Geometry: final body of the model. Coordinates: model frame, mm. A direction names the side the tool comes from. Round coordinates to 2 decimals unless told otherwise and drop trailing zeros. Loops run counter-clockwise (first coordinate to the right, second up) from the corner with the lowest first, then second, coordinate; pieces in that order, holes last. Notation, with made-up numbers: M -5,89.25 L 49,89.25 A20 ccw 49,122.25 Z; hole C 71.25,-36 d7. An arc over 180 degrees is marked long. Answer as a JSON object with one key per item and string values.
Autodesk Inventor part; units mm, degrees
ref_plane "YZ Plane" through (0, 0, 0) normal (1, 0, 0) x (0, 1, 0)
ref_plane "XZ Plane" through (0, 0, 0) normal (0, 1, 0) x (-1, 0, 0)
ref_plane "XY Plane" through (0, 0, 0) normal (0, 0, 1) x (1, 0, 0)
sketch "Sketch1" plane through (0, 0, 0) normal (0, 0, 1) x (1, 0, 0)
  line L0 (0, 0) -> (10, 0)
  line L1 (10, 0) -> (10, 10)
  line L2 (10, 10) -> (0, 10)
  line L3 (0, 10) -> (0, 0)
  dimension "d0" = 10
  dimension "d1" = 10
extrude "Extrusion1" add sketch "Sketch1" along normal blind 1
sketch "Sketch2" plane through (0, 0, 1) normal (0, 0, 1) x (1, 0, 0)
  line L0 (10, 10) -> (0, 10)
  line L1 (5, 10) -> (5, 5)
  circle A0 centre (5, 5) radius 3.25
  point P0 (0, 0)
  dimension "d4" = 5
  dimension "d5" = 6.5
extrude "Extrusion2" add sketch "Sketch2" along normal blind 0.5
sketch "Sketch3" plane through (5, 5, 1.5) normal (0, 0, 1) x (1, 0, 0)
  circle A0 centre (0, 0) radius 3
  point P0 (-5, -5)
  dimension "d8" = 6
extrude "Extrusion3" add sketch "Sketch3" along normal blind 0.5
sketch "Sketch4" plane through (5, 5, 2) normal (0, 0, 1) x (1, 0, 0)
  line L0 (1, 0) -> (1, 1)
  line L1 (1, 1) -> (-1, 1)
  line L2 (-1, 1) -> (-1, -1)
  line L3 (-1, -1) -> (1, -1)
  line L4 (1, -1) -> (1, 0)
  point P0 (-5, -5)
  dimension "d12" = 1
  dimension "d13" = 2
  dimension "d14" = 2
extrude "Extrusion4" add sketch "Sketch4" along normal blind 2.5
sketch "Sketch5" plane through (0, 0, 1) normal (0, 0, 1) x (1, 0, 0)
  point P0 (0, 0)
sketch "Sketch6" plane through (5, 5, 4.5) normal (0, 0, 1) x (1, 0, 0)
  point P0 (-5, -5)
properties part number "BTN_2"
1) Pin query (flat end, axial travel): P1, Ø1.6, axis at x = 4.5, z = 2.5, coming from the -Y side; P2, Ø1, axis at y = 5.5, z = 3, coming from the -X side; P3, Ø4, axis at x = 2, y = 8.5, coming from the +Z side. Return the tip coordinate at first contact, or that it passes through.
Results:
{"P1": "y = 2", "P2": "x = 4", "P3": "z = 2"}
2) Ray query, line 1 (Z direction, x = 0.5, y = 7.25); line 2 (Z direction, x = 6.5, y = 4.5); line 3 (X direction, y = 4.75, z = 2.1). Return the intervals inside material, ascending.
Results:
{"line 1": "0 to 1", "line 2": "0 to 2", "line 3": "4 to 6"}
3) Section query A-A (y = 5). Return the cut outline in (x, z), and give its area (4 significant figures).
Results:
{"outline": "M 0,0 L 10,0 L 10,1 L 8.25,1 L 8.25,1.5 L 8,1.5 L 8,2 L 6,2 L 6,4.5 L 4,4.5 L 4,2 L 2,2 L 2,1.5 L 1.75,1.5 L 1.75,1 L 0,1 Z", "area": "21.25 mm2"}
4) Reachability of faces 1 (the flat face through (6, 5, 3)), 2 (the flat face through (5, 4, 3)), 3 (the flat face through (4, 5, 3)), 4 (the flat face through (1.6, 5.1, 1)) from +Z, -Z, +X, -X, +Y, -Y: full face, straight path, thin tool, end or side. Return the list, or none.
Results:
{"face 1": "+Z, +X, +Y, -Y", "face 2": "+Z, +X, -X, -Y", "face 3": "+Z, -X, +Y, -Y", "face 4": "+Z"}
5) Section query C-C (z = 4.05). Return the cut outline in (x, y).
Results:
{"outline": "M 4,4 L 6,4 L 6,6 L 4,6 Z"}
6) Section query D-D (x = 3.5). Return the cut outline in (y, z), and give its area (3 significant figures).
Results:
{"outline": "M 0,0 L 10,0 L 10,1 L 7.88,1 L 7.88,1.5 L 7.6,1.5 L 7.6,2 L 2.4,2 L 2.4,1.5 L 2.12,1.5 L 2.12,1 L 0,1 Z", "area": "15.5 mm2"}
